from build123d import *

# Parameters (mm, degrees)
BOSS_EXTRUDE1_DEPTH      = 24
CUT_EXTRUDE1_DEPTH       = 48
CUT_EXTRUDE2_DEPTH       = 19
CUT_EXTRUDE3_DEPTH       = 42.036569057
CHAMFER1_SIZE            = 2.3
SKETCH6_W                = 20.5
SKETCH6_H                = 23
CUT_EXTRUDE4_DEPTH       = 2.5
SKETCH7_R                = 2.5
BOSS_EXTRUDE2_DEPTH      = 2.5
CUT_EXTRUDE5_DEPTH       = 44.462627624
CHAMFER1_OF_MIRROR1_SIZE = 2.3


with BuildPart() as part:
    # Sketch1 → Boss-Extrude1 (new, symmetric)
    with BuildSketch(Plane(origin=(0, 0, 0), x_dir=(0, 0, -1), z_dir=(1, 0, 0))):
        with BuildLine():
            Line((16.5, -11.5), (-16.5, -11.5))
            ThreePointArc((-16.5, -11.5), (-28, 0), (-16.5, 11.5))
            Line((-16.5, 11.5), (16.5, 11.5))
            Line((16.5, 11.5), (16.5, -11.5))
        make_face()
    extrude(amount=BOSS_EXTRUDE1_DEPTH, both=True)

    # Sketch2 → Cut-Extrude1 (cut)
    with BuildSketch(Plane(origin=(24, 0, 0), x_dir=(0, 0, -1), z_dir=(1, 0, 0))):
        Polygon((16.5, 0), (-3.5, 11.5), (16.5, 11.5), align=None)
    extrude(amount=-CUT_EXTRUDE1_DEPTH, mode=Mode.SUBTRACT)

    # Sketch4 → Cut-Extrude2 (cut, symmetric)
    with BuildSketch(Plane(origin=(0, 0, 0), x_dir=(0, 0, -1), z_dir=(1, 0, 0))):
        with BuildLine():
            Line((16.5, -6.5), (16.5, 0))
            Line((16.5, 0), (-3.5, 11.5))
            Line((-3.5, 11.5), (-16.5, 11.5))
            ThreePointArc((-16.5, 11.5), (-28, 0), (-16.5, -11.5))
            Line((-16.5, -11.5), (-7.5, -11.5))
            Line((-7.5, -11.5), (-7.5, -9.5))
            Line((-7.5, -9.5), (-1.339824897, -9.5))
            Line((-1.339824897, -9.5), (2.5, -6.5))
            Line((2.5, -6.5), (16.5, -6.5))
        make_face()
    extrude(amount=CUT_EXTRUDE2_DEPTH, both=True, mode=Mode.SUBTRACT)

    # Sketch5 → Cut-Extrude3 (cut, through all)
    with BuildSketch(Plane(origin=(0, -6.5, 0), x_dir=(1, 0, 0), z_dir=(0, 1, 0))):
        with BuildLine():
            Line((6.5, 11.5), (12.5, 11.5))
            ThreePointArc((12.5, 11.5), (14.5, 9.5), (12.5, 7.5))
            Line((12.5, 7.5), (6.5, 7.5))
            ThreePointArc((6.5, 7.5), (4.5, 9.5), (6.5, 11.5))
        make_face()
    cut_extrude3 = extrude(amount=-CUT_EXTRUDE3_DEPTH, mode=Mode.SUBTRACT)

    # Chamfer1
    chamfer1_edges = [part.edges().sort_by_distance(p)[0] for p in [
        (4.5, -6.5, -9.5),
        (9.5, -6.5, -7.5),
        (14.5, -6.5, -9.5),
        (9.5, -6.5, -11.5),
    ]]
    chamfer(chamfer1_edges, length=CHAMFER1_SIZE)

    # Sketch6 → Cut-Extrude4 (cut)
    with BuildSketch(Plane(origin=(24, 0, 0), x_dir=(0, 0, -1), z_dir=(1, 0, 0))):
        with Locations((-17.75, 0)):
            Rectangle(SKETCH6_W, SKETCH6_H)
    cut_extrude4 = extrude(amount=-CUT_EXTRUDE4_DEPTH, mode=Mode.SUBTRACT)

    # Sketch7 → Boss-Extrude2 (add)
    with BuildSketch(Plane(origin=(21.5, 0, 0), x_dir=(0, 0, -1), z_dir=(1, 0, 0))):
        with Locations(Location((-16.5, 0, 0), (0, 0, 180))):
            Circle(SKETCH7_R)
    boss_extrude2 = extrude(amount=BOSS_EXTRUDE2_DEPTH)

    # Sketch8 → Cut-Extrude5 (cut, through all)
    with BuildSketch(Plane(origin=(0, 11.5, 0), x_dir=(1, 0, 0), z_dir=(0, 1, 0))):
        Polygon((24, -16.5), (22.75, -19), (24, -19), align=None)
    extrude(amount=-CUT_EXTRUDE5_DEPTH, mode=Mode.SUBTRACT)

    # Mirror1: Cut-Extrude3, Cut-Extrude4, Boss-Extrude2 across plane
    add(cut_extrude3.mirror(Plane(origin=(0, 0, 0), x_dir=(0, 0, 1), z_dir=(1, 0, 0))), mode=Mode.SUBTRACT)
    add(cut_extrude4.mirror(Plane(origin=(0, 0, 0), x_dir=(0, 0, 1), z_dir=(1, 0, 0))), mode=Mode.SUBTRACT)
    add(boss_extrude2.mirror(Plane(origin=(0, 0, 0), x_dir=(0, 0, 1), z_dir=(1, 0, 0))))

    # Chamfer1 of Mirror1
    chamfer1_of_mirror1_edges = [part.edges().sort_by_distance(p)[0] for p in [
        (-4.5, -6.5, -9.5),
        (-9.5, -6.5, -7.5),
        (-14.5, -6.5, -9.5),
        (-9.5, -6.5, -11.5),
    ]]
    chamfer(chamfer1_of_mirror1_edges, length=CHAMFER1_OF_MIRROR1_SIZE)


solid = part.part
Could you check a few things on this model? Use its own coordinates, in mm. A direction names the side the tool comes from. Give positions to 0.01 mm unless a question says otherwise; leave off trailing zeros. Order: outer loops, then holes, each group sorted by start corner. A loop starts at its lowest first (then second) coordinate and runs counter-clockwise, first axis right, second up.
Item 1: If we section it at C-C, the plane y = -5: Write out the boundary of the cut face in (x, z).
Item 2: If we section it at D-D, the plane z = 23: Write out the boundary of the cut face in (x, y), plus the area to 3 significant figures.
Item 3: I need wall thicknesses on line 1 (X direction, y = 10.25, z = 8); line 2 (X direction, y = -1.25, z = -14); line 3 (Z direction, x = 16.5, y = -9.75). Which ranges of each line are inside material? Lowest first, please.
Item 4: I'm going to push flat-ended pins straight in: pin 1 (2 mm diameter, centred on x = -23, y = -5.5, fed in from +Z); pin 2 (1.5 mm diameter, centred on y = 7, z = 19.5, fed in from +X); pin 3 (1.5 mm diameter, centred on x = -0.5, y = -6.5, fed in from +Z). Where does each tip first touch, or does it pass through?
Item 5: If we mould it in two halves opening along Z, with no side actions, what happens to faces 5 (the face through (20, 0, 28)), 6 (the face through (-24, 0, 16)), 7 (the face through (4.5, -10.1, -9.5))? For each: pulls with the +Z half, pulls with the -Z half, needs draft (parallel to the pull), parting line crosses it, or undercut.
Item 6: If we section it at B-B, the plane z = -9.5: Write out the boundary of the cut face in (x, y) (3 decimals).
Item 7: For faces 1 (the face through (-3.9, -8.2, -9.4)), 2 (the face through (0.266, -8.021, -0.553)), 3 (the face through (-23, 0, 7.5)), 4 (the face through (-23, 0, 14)), which set-ups out of +Z, -Z, +X, -X, +Y, -Y let a thin tool reach every point of the face, with its end or its side?
Item 8: If we section it at A-A, the plane z = 9: Write out the boundary of the cut face in (x, y), plus the area to 3 significant figures.
Values:
1. outline: (-24, -16.5) - (-19, -16.5) - (-19, 26.86) - (-21.5, 26.86) - (-21.5, 7.5) - (-24, 7.5) - close; (19, -16.5) - (24, -16.5) - (24, 7.5) - (21.5, 7.5) - (21.5, 26.86) - (19, 26.86) - close
2. outline: (-21.5, -9.49) - (-19, -9.49) - (-19, 9.49) - (-21.5, 9.49) - close; (19, -9.49) - (21.5, -9.49) - (21.5, 9.49) - (19, 9.49) - close
2. area: 94.9 mm2
3. line 1: x = -21.5 to -19, 19 to 21.5
3. line 2: x = -24 to -19, 19 to 24
3. line 3: z = -16.5 to 7.5
4. pin 1: stops at z = 7.5
4. pin 2: stops at x = 21.5
4. pin 3: stops at z = -1.54
5. face 5: pulls with the +Z half
5. face 6: needs draft
5. face 7: undercut
6. outline: (-24, -11.5) - (-14.5, -11.5) - (-14.5, -8.8) - (-16.8, -6.5) - (-19, -6.5) - (-19, 4.025) - (-24, 4.025) - close; (-4.5, -11.5) - (4.5, -11.5) - (4.5, -8.8) - (2.2, -6.5) - (-2.2, -6.5) - (-4.5, -8.8) - close; (14.5, -11.5) - (24, -11.5) - (24, 4.025) - (19, 4.025) - (19, -6.5) - (16.8, -6.5) - (14.5, -8.8) - close
7. face 1: +Y
7. face 2: +Z, +Y
7. face 3: -X, +Y, -Y
7. face 4: -X
8. outline: (-21.5, -11.5) - (-19, -11.5) - (-19, 11.5) - (-21.5, 11.5) - close; (19, -11.5) - (21.5, -11.5) - (21.5, 11.5) - (19, 11.5) - close
8. area: 115 mm2
